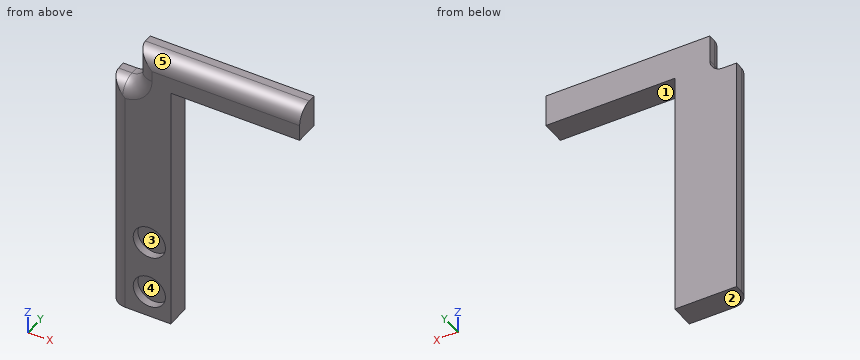
```python
from build123d import *

# Parameters (mm, degrees)
EXTRUDE_1_DEPTH     = 9
FILLET_1_R          = 6
SKETCH_2_R          = 6
CUT_EXTRUDE_1_DEPTH = 3


with BuildPart() as part:
    # 草圖1 → 填料-伸長1 (new body)
    with BuildSketch(Plane(origin=(0, 0, 0), x_dir=(1, 0, 0), z_dir=(0, 1, 0))):
        with BuildLine():
            Line((0, 0), (-48, 0))
            Line((-48, 0), (-48, 94))
            Line((-48, 94), (-71, 94))
            Line((-71, 94), (-71, 3))
            Line((-71, 3), (-66, 3))
            ThreePointArc((-66, 3), (-62.464466094, 1.535533906), (-61, -2))
            Line((-61, -2), (-61, -12))
            Line((-61, -12), (0, -12))
            Line((0, -12), (0, 0))
        make_face()
    extrude(amount=EXTRUDE_1_DEPTH)

    # 圓角1
    # the kernel refuses this fillet: 6 mm, written as the material it takes off along each edge
    with BuildSketch(Plane(origin=(-76, 0, 12), x_dir=(0, 1, 0), z_dir=(1, 0, 0))) as fillet_1_piece_1:
        with BuildLine():
            CenterArc((FILLET_1_R, -FILLET_1_R), FILLET_1_R, 90, 90)
            Line((0, -FILLET_1_R), (0, 0))
            Line((0, 0), (FILLET_1_R, 0))
        make_face()
    extrude(amount=91, mode=Mode.SUBTRACT)
    with BuildSketch(Plane(origin=(-61, 0, 2), x_dir=(0, 1, 0), z_dir=(0, 0, 1))) as fillet_1_piece_2:
        with BuildLine():
            CenterArc((FILLET_1_R, -FILLET_1_R), FILLET_1_R, 90, 90)
            Line((0, -FILLET_1_R), (0, 0))
            Line((0, 0), (FILLET_1_R, 0))
        make_face()
    extrude(amount=25, mode=Mode.SUBTRACT)
    with BuildSketch(Plane(origin=(-66, 0, 2), x_dir=(0, 0, -1), z_dir=(-1, 0, 0))) as fillet_1_piece_3:
        with BuildLine():
            CenterArc((5 + FILLET_1_R, -FILLET_1_R), FILLET_1_R, 90, 90)
            Line((5 + FILLET_1_R, 0), (5, 0))
            Line((5, 0), (5, -FILLET_1_R))
        make_face()
    revolve(axis=Axis((-66, 0, 2), (0, -1, 0)), revolution_arc=90, mode=Mode.SUBTRACT)
    with BuildSketch(Plane(origin=(-71, 0, -109), x_dir=(0, 1, 0), z_dir=(0, 0, 1))) as fillet_1_piece_4:
        with BuildLine():
            CenterArc((FILLET_1_R, -FILLET_1_R), FILLET_1_R, 90, 90)
            Line((0, -FILLET_1_R), (0, 0))
            Line((0, 0), (FILLET_1_R, 0))
        make_face()
    extrude(amount=121, mode=Mode.SUBTRACT)
    with BuildSketch(Plane(origin=(-86, 0, -3), x_dir=(0, 1, 0), z_dir=(1, 0, 0))) as fillet_1_piece_5:
        with BuildLine():
            CenterArc((FILLET_1_R, -FILLET_1_R), FILLET_1_R, 90, 90)
            Line((0, -FILLET_1_R), (0, 0))
            Line((0, 0), (FILLET_1_R, 0))
        make_face()
    extrude(amount=20, mode=Mode.SUBTRACT)

    # 草圖2 → 除料-伸長1 (cut)
    with BuildSketch(Plane.XZ):
        with Locations(Location((-56, -84, 0), (0, 0, 270))):
            Circle(SKETCH_2_R)
        with Locations(Location((-56, -64, 0), (0, 0, 270))):
            Circle(SKETCH_2_R)
    extrude(amount=-CUT_EXTRUDE_1_DEPTH, mode=Mode.SUBTRACT)


solid = part.part
```
Build history of the part. All positions in model axes, mm. Face numbers are marked on the shaded views. A direction names the side the tool comes from. Round coordinates to 2 decimals unless told otherwise and drop trailing zeros. Loops run counter-clockwise (first coordinate to the right, second up) from the corner with the lowest first, then second, coordinate; pieces in that order, holes last.
Item 1: Saw through at A-A (y = 7.5). List the corners of the cut face in (x, z).
Item 2: Saw through at B-B (z = -84). List the corners of the cut face in (x, y), then the cut area to 3 significant figures.
Item 3: Saw through at D-D (y = 1.75). List the corners of the cut face in (x, z), then the cut area to 3 significant figures.
Item 4: Saw through at C-C (x = -53). List the corners of the cut face in (y, z), then the cut area to 3 significant figures.
Item 5: Which spindle directions (+Z, -Z, +X, -X, +Y, -Y) get a long thin tool onto all of the face, cutting with end or side? Do the marked faces 1, 2 and 3. Say none if no direction does.
Item 6: Drill centre lines: line 1 along X through (y, z) = (7.25, -58); line 2 along Y through (x, z) = (-66, -41); line 3 along X through (y, z) = (2, -84). Where is each one in solid material? Low to high.
Item 7: Two-plate mould, pull along X, no slides. Class the marked faces 4 and 5: released by +X, released by -X, zero draft, split by the parting line, or undercut.
Item 8: Pin check, flat tips, straight feed: P1, Ø6, axis at x = -58.5, z = -63.5, coming from the -Y side; P2, Ø1, axis at x = -14, y = 4.5, coming from the -Z side; P3, Ø2.5, axis at y = 5, z = -60.5, coming from the +X side; P4, Ø4, axis at y = 5, z = -31, coming from the -X side. Stop position of each tip, or through.
Worked answers:
1. outline: (-71, -94) - (-48, -94) - (-48, 0) - (0, 0) - (0, 12) - (-61, 12) - (-61, 2) arc R5 cw to (-66, -3) - (-71, -3) - close
2. outline: (-71, 6) arc R6 ccw to (-65, 0) - (-62, 0) - (-62, 3) - (-50, 3) - (-50, 0) - (-48, 0) - (-48, 9) - (-71, 9) - close
2. area: 163 mm2
3. outline: (-69.24, -94) - (-48, -94) - (-48, 0) - (0, 0) - (0, 10.24) - (-59.24, 10.24) - (-59.24, 2) arc R6.76 cw to (-66, -4.76) - (-69.24, -4.76) - close; hole circle Ø12 at (-56, -84); hole circle Ø12 at (-56, -64)
3. area: 2,340 mm2
4. outline: (0, -94) - (9, -94) - (9, 12) - (6, 12) arc R6 ccw to (0, 6) - (0, -58.8) - (3, -58.8) - (3, -69.2) - (0, -69.2) - (0, -78.8) - (3, -78.8) - (3, -89.2) - (0, -89.2) - close
4. area: 884 mm2
5. face 1: -Z, +X, +Y, -Y
5. face 2: -Z, +X, -X, +Y, -Y
5. face 3: -Y
6. line 1: x = -71 to -48
6. line 2: y = 0.08 to 9
6. line 3: x = -69.47 to -62, -50 to -48
7. face 4: undercut
7. face 5: zero draft
8. P1: stops at y = 3
8. P2: stops at z = 0
8. P3: stops at x = -48
8. P4: stops at x = -71
